from build123d import *

# Parameters (mm, degrees)
BOSS_EXTRUDE1_REACH     = 69.5
BOSS_EXTRUDE1_START     = 25
SKETCH2_R               = 18
BOSS_EXTRUDE2_REACH     = 69.5
BOSS_EXTRUDE2_START     = -25
SKETCH2_2_R             = 18
SKETCH3_R               = 11
CUT_EXTRUDE1_DEPTH      = 43.5
CUT_EXTRUDE1_DEPTH_BACK = 43.5


with BuildPart() as part:
    # Sketch1 → Revolve1 (revolve)
    with BuildSketch(Plane.XY):
        with BuildLine():
            Line((42.5, 7), (42.5, 5))
            Line((42.5, 5), (38.5, 5))
            Line((38.5, 5), (38.5, 2))
            Line((38.5, 2), (42.5, 2))
            Line((42.5, 2), (42.5, 0))
            Line((42.5, 0), (38.5, 0))
            Line((38.5, 0), (38.5, -3))
            Line((38.5, -3), (42.5, -3))
            Line((42.5, -3), (42.5, -5))
            Line((42.5, -5), (38.5, -5))
            Line((38.5, -5), (38.5, -8))
            Line((38.5, -8), (42.5, -8))
            Line((42.5, -8), (42.5, -10))
            Line((42.5, -10), (38.5, -10))
            Line((38.5, -10), (38.5, -13))
            Line((38.5, -13), (42.5, -13))
            Line((42.5, -13), (42.5, -60))
            Line((42.5, -60), (38.5, -60))
            Line((38.5, -60), (38.5, -62))
            Line((38.5, -62), (42.5, -62))
            Line((42.5, -62), (42.5, -67))
            Line((42.5, -67), (37, -67))
            Line((37, -67), (37, 0))
            Line((37, 0), (0, 0))
            Line((0, 0), (0, 11.840422459))
            ThreePointArc((0, 11.840422459), (21.387377642, 10.626417884), (42.5, 7))
        make_face()
    revolve(axis=Axis((0, 0, 0), (0, 1, 0)))

    # Sketch2 → Boss-Extrude1 (add, up to next)
    with BuildSketch(Plane.XY.offset(BOSS_EXTRUDE1_START), mode=Mode.PRIVATE) as boss_extrude1_sk1:
        with Locations((0, -40)):
            Circle(SKETCH2_R)
    boss_extrude1_tool1 = extrude(boss_extrude1_sk1.sketch, amount=BOSS_EXTRUDE1_REACH, mode=Mode.PRIVATE) - part.part
    add(boss_extrude1_tool1.solids().sort_by_distance((0, -40, 25))[0])

    # Sketch2<2> → Boss-Extrude2 (add, up to next)
    with BuildSketch(Plane.XY.offset(BOSS_EXTRUDE2_START), mode=Mode.PRIVATE) as boss_extrude2_sk1:
        with Locations((0, -40)):
            Circle(SKETCH2_2_R)
    boss_extrude2_tool1 = extrude(boss_extrude2_sk1.sketch, amount=-BOSS_EXTRUDE2_REACH, mode=Mode.PRIVATE) - part.part
    add(boss_extrude2_tool1.solids().sort_by_distance((0, -40, -25))[0])

    # Sketch3 → Cut-Extrude1 (cut, two sides)
    with BuildSketch(Plane.XY) as cut_extrude1_sk:
        with Locations((0, -40)):
            Circle(SKETCH3_R)
    extrude(amount=CUT_EXTRUDE1_DEPTH, mode=Mode.SUBTRACT)
    extrude(cut_extrude1_sk.sketch, amount=-CUT_EXTRUDE1_DEPTH_BACK, mode=Mode.SUBTRACT)


solid = part.part
The listing builds one solid part. Answer for the finished solid, in the listing's coordinates (mm). A direction names the side the tool comes from. Round coordinates to 2 decimals unless told otherwise and drop trailing zeros. Write each loop counter-clockwise with the first axis right and the second up, starting at its lowest first coordinate (ties: lowest second). Pieces come first, ordered by that corner, then holes. Notation, with made-up numbers: M 31.25,-40 L 89.25,-40 A20 cw 89.25,-15 Z; hole C 85.25,8.5 d3. An arc over 180 degrees is marked long. Write each question's results on one line, items separated by ' | '. Start each with the question number.
(1) Each of these flat-tipped pins is pushed along its axis until it touches: P1, Ø5, axis at x = -8, y = -21, coming from the +Z side; P2, Ø3, axis at y = -26, z = -22, coming from the +X side; P3, Ø6, axis at y = -5, z = 26.5, coming from the +X side; P4, Ø13, axis at x = 0, y = -40, coming from the -Z side. Where does it stop, or does it pass through?
(2) For faces 4 (the cylindrical face through (-33.727, -9.014, 25.861)), 5 (the flat face through (-8, -48, 25)), 6 (the cylindrical face through (-30.55, -11.52, 23.43)), determine the directions among +Z, -Z, +X, -X, +Y, -Y from which every point of the face is accessible in a straight line to the end or side of a thin tool.
(3) The part is cut by section B-B, the plane x = 0. Give the number of separate pieces and of enclosed holes in the cut face, and give its area (3 significant figures).
(4) Determine the mould class of faces 1 (the cylindrical face through (-30.55, -6.52, 23.43)), 2 (the cylindrical face through (-33.727, 5.986, 25.861)), 3 (the cylindrical face through (-17.983, -39.209, -29.583)) for opening direction Y: +Y half, -Y half, draft (parallel to the pull), parting line (faces both ways), or undercut.
(5) The part is cut by section A-A, the plane y = -40. Write down the section's boundary in (x, z), and give its area (3 significant figures).
(6) The part is cut by section C-C, the plane y = -15. Write down the section's boundary in (x, z), and give its area (3 significant figures).
(7) Find the intervals of material crossed by line 1 (Y direction, x = 0, z = 36); line 2 (Y direction, x = -31, z = 23); line 3 (Y direction, x = 0, z = 34), in increasing order.
Worked answers:
1) P1: stops at z = 42.14 | P2: stops at x = 37.23 | P3: stops at x = 35.41 | P4: passes through
2) face 4: +Y, -Y | face 5: -Y | face 6: none
3) separate pieces: 3 | enclosed holes: 0 | area: 1,590 mm²
4) face 1: undercut | face 2: draft | face 3: undercut
5) outline: M -18,-32.33 A37 cw -18,32.33 L -18,25 L -11,25 L -11,41.05 A42.5 ccw -11,-41.05 L -11,-25 L -18,-25 Z; M 11,-41.05 A42.5 ccw 11,41.05 L 11,25 L 18,25 L 18,32.33 A37 cw 18,-32.33 L 18,-25 L 11,-25 Z | area: 1,380 mm²
6) outline: C 0,0 d85; hole C 0,0 d74 | area: 1,370 mm²
7) line 1: y = -58 to -51, -29 to -22, 0 to 8.38 | line 2: y = -67 to -62, -60 to -13, -10 to -8, -5 to -3, 0 to 2, 5 to 7.86 | line 3: y = -58 to -51, -29 to -22, 0 to 8.76
